```python
from build123d import *

# Parameters (mm, degrees)
ESBO_O1_R                = 2
RESSALTO_EXTRUS_O1_DEPTH = 2.25
CHANFRO1_SIZE            = 0.5
FILETE1_R                = 0.5


with BuildPart() as part:
    # Esboço1 → Ressalto-extrusão1 (new, symmetric)
    with BuildSketch(Plane(origin=(0, 0, 0), x_dir=(1, 0, 0), z_dir=(0, 1, 0))):
        with BuildLine():
            Line((-26, 4), (26, 4))
            ThreePointArc((26, 4), (30, 0), (26, -4))
            Line((26, -4), (-26, -4))
            ThreePointArc((-26, -4), (-30, 0), (-26, 4))
        make_face()
        with Locations(Location((0, 0, 0), (0, 0, 270))):
            Circle(ESBO_O1_R, mode=Mode.SUBTRACT)
        with BuildLine():
            Line((26, -2), (22, -2))
            ThreePointArc((22, -2), (20, 0), (22, 2))
            Line((22, 2), (26, 2))
            ThreePointArc((26, 2), (28, 0), (26, -2))
        make_face(mode=Mode.SUBTRACT)
    extrude(amount=RESSALTO_EXTRUS_O1_DEPTH, both=True)

    # Chanfro1
    chanfro1_edges = [part.edges().sort_by_distance(p)[0] for p in [
        (0, -2.25, -2),
        (0, 2.25, -2),
        (28, -2.25, 0),
        (24, -2.25, -2),
        (20, -2.25, 0),
        (24, -2.25, 2),
        (28, 2.25, 0),
        (24, 2.25, -2),
        (20, 2.25, 0),
        (24, 2.25, 2),
    ]]
    chamfer(chanfro1_edges, length=CHANFRO1_SIZE)

    # Filete1
    filete1_edges = [part.edges().sort_by_distance(p)[0] for p in [
        (30, 2.25, 0),
        (0, 2.25, -4),
        (-30, 2.25, 0),
        (0, -2.25, -4),
        (30, -2.25, 0),
        (0, -2.25, 4),
        (-30, -2.25, 0),
        (0, 2.25, 4),
    ]]
    fillet(filete1_edges, radius=FILETE1_R)


solid = part.part
```
For this review, take the finished solid that the model builds, in its own axes (mm). A direction names the side the tool comes from. Round coordinates to 2 decimals unless told otherwise and drop trailing zeros. Write each loop counter-clockwise with the first axis right and the second up, starting at its lowest first coordinate (ties: lowest second). Pieces come first, ordered by that corner, then holes. Notation, with made-up numbers: M 14,-7 L 63,-7 A16 cw 63,13 Z; hole C 27.5,49 d8. An arc over 180 degrees is marked long. One line per item, written item: value. Start each with the question number.
(1) Wall thickness on line 1 (X direction, y = 0, z = 0); line 2 (X direction, y = 1.55, z = -1.5); line 3 (Z direction, x = 14, y = 1.9): over which ranges is each line inside the solid? List them lowest first.
(2) Insertion check: pin 1 (1 mm diameter, centred on y = 0, z = -1.5, fed in from -X); pin 2 (1 mm diameter, centred on y = -1, z = -1.5, fed in from +X). Each pin has a flat end and moves straight along its axis. Give the tip position at first contact, or say it passes through.
(3) We need section C-C (z = -0.75). Count the separate pieces of the cut face and the enclosed holes in it, and give its area (3 significant figures).
(4) We need section B-B (y = 0). Give the boundary of the cut face in (x, z), and give its area (3 significant figures).
(5) We need section A-A (x = 0). Give the boundary of the cut face in (y, z).
(6) The part is to be moulded in two halves that separate along X. For faces 5 (the cylindrical face through (-30, 0, 0)), 6 (the conical face through (19.865, 1.885, 0.047)), 7 (the flat face through (0, 0, -4)), say which applies: released by +X, released by -X, zero draft, split by the parting line, or undercut.
(7) Machinability: for faces 1 (the cylindrical face through (20, 0, 0)), 2 (the conical face through (28.135, 1.885, -0.047)), 3 (the flat face through (-6, 2.25, 0)), 4 (the conical face through (19.86, -1.89, 0.05)), which of the approach directions +Z, -Z, +X, -X, +Y, -Y give a long, thin tool a straight path to every point of the face, cutting with its end or side? Answer none if there is none.
Result:
1. line 1: -30 to -2, 2 to 20, 28 to 30
1. line 2: -29.71 to -1.32, 1.32 to 20.68, 27.32 to 29.71
1. line 3: -3.98 to 3.98
2. pin 1: x = -29.87
2. pin 2: x = 29.87
3. separate pieces: 3
3. enclosed holes: 0
3. area: 217 mm²
4. outline: M -26,-4 L 26,-4 A4 ccw 26,4 L -26,4 A4 ccw Z; hole C 0,0 d4; hole M 22,-2 L 26,-2 A2 ccw 26,2 L 22,2 A2 ccw Z
4. area: 425 mm²
5. outline: M -2.25,-3.5 A0.5 ccw -1.75,-4 L 1.75,-4 A0.5 ccw 2.25,-3.5 L 2.25,-2.5 L 1.75,-2 L -1.75,-2 L -2.25,-2.5 Z; M -2.25,2.5 L -1.75,2 L 1.75,2 L 2.25,2.5 L 2.25,3.5 A0.5 ccw 1.75,4 L -1.75,4 A0.5 ccw -2.25,3.5 Z
6. face 5: released by -X
6. face 6: undercut
6. face 7: zero draft
7. face 1: +Y, -Y
7. face 2: +Y
7. face 3: +Z, -Z, +X, -X, +Y
7. face 4: -Y
